Read the model definition and answer for the solid it produces. Units are mm, in the model's axes. Coordinates: 2 decimals unless noted, no trailing zeros. Loops run counter-clockwise (first coordinate to the right, second up) from the corner with the lowest first, then second, coordinate; pieces in that order, holes last. Notation, with made-up numbers: M 57,89 L 100,89 A25 cw 100,118 Z; hole C 81,9.25 d8. An arc over 180 degrees is marked long. Put each result on its own line as item: value.
from build123d import *

# Parameters (mm, degrees)
F0_R     = 15
F1_DEPTH = 50
F2_D     = 22
F4_D     = 5.8
F4_DEPTH = 15.001


with BuildPart() as f1:
    # F0 (on Top) → F1 (new body)
    with BuildSketch(Plane.XY):
        Circle(F0_R)
    extrude(amount=F1_DEPTH)

    # F2 (through all)
    with Locations(Plane(origin=(0, 0, 0), x_dir=(1, 0, 0), z_dir=(0, 0, -1))):
        with Locations((0, 0)):
            Hole(F2_D / 2)

    # F4 (through all, one way)
    with BuildSketch(Plane.YZ):
        with Locations((0, 25)):
            Circle(F4_D / 2)
    extrude(amount=-F4_DEPTH, mode=Mode.SUBTRACT)


solid = f1.part
1) Find section D-D, the plane y = 7. Write down the section's boundary in (x, z), plus the area to 3 significant figures.
Answer list:
outline: M -13.27,0 L -8.49,0 L -8.49,50 L -13.27,50 Z; M 8.49,0 L 13.27,0 L 13.27,50 L 8.49,50 Z
area: 478 mm^2
2) Find section B-B, the plane x = 0. Write down the section's boundary in (y, z), plus the area to 3 significant figures.
Answer list:
outline: M -15,0 L -11,0 L -11,50 L -15,50 Z; M 11,0 L 15,0 L 15,50 L 11,50 Z
area: 400 mm^2
3) Given pin 1 Ø5 at (y, z) = (-6, 35.5) entering from -X; pin 2 Ø2 at (x, z) = (12, 11) entering from +Y; pin 3 Ø3.5 at (y, z) = (0, 25) entering from -X, each flat-ended and moving along its own axis, determine where each tip first touches the part or whether it passes through.
Answer list:
pin 1: stops at x = -14.59
pin 2: stops at y = 10.2
pin 3: stops at x = 10.86
4) Find section C-C, the plane z = 21.5. Write down the section's boundary in (x, y).
Answer list:
outline: C 0,0 d30; hole C 0,0 d22
5) Straight lines are drawn through the part: line 1 (Y direction, x = 0, z = 33); line 2 (X direction, y = -6, z = 6); line 3 (X direction, y = 5.5, z = 29). For each, find the intervals that lie inside material, in ascending order. Write a range as [from, to].
Answer list:
line 1: y = [-15, -11], [11, 15]
line 2: x = [-13.75, -9.22], [9.22, 13.75]
line 3: x = [-13.96, -9.53], [9.53, 13.96]
6) Find section A-A, the plane y = 0. Write down the section's boundary in (x, z).
Answer list:
outline: M -15,0 L -11,0 L -11,22.1 L -15,22.1 Z; M -15,27.9 L -11,27.9 L -11,50 L -15,50 Z; M 11,0 L 15,0 L 15,50 L 11,50 Z
7) Determine the mould class of faces 1 (the flat face through (-5, 10, 0)), 2 (the cylindrical face through (2.38, 10.74, 25.35)), 3 (the cylindrical face through (-12.78, 2.68, 23.89)) for opening direction Z: released by +Z, released by -Z, zero draft, split by the parting line, or undercut.
Answer list:
face 1: released by -Z
face 2: zero draft
face 3: undercut
